```python
from build123d import *

# Parameters (mm, degrees)
SKETCH080_W         = 21.5
SKETCH080_H         = 41.5
PAD036_DEPTH        = 7
SKETCH081_W         = 17.5
SKETCH081_H         = 37.5
POCKET027_DEPTH     = 5
SKETCH077_W         = 13.5
SKETCH077_H         = 33.5
POCKET028_DEPTH     = 2.001
SKETCH078_W         = 13.5
SKETCH078_H         = 4
POCKET026_DEPTH     = 7.001
REVOLUTION010_ANGLE = -180
REVOLUTION011_ANGLE = -180


with BuildPart() as part:
    # Sketch080 → Pad036 (new body)
    with BuildSketch(Plane.XY):
        with Locations((10.75, 20.75)):
            Rectangle(SKETCH080_W, SKETCH080_H)
    extrude(amount=PAD036_DEPTH)

    # Sketch081 (on Face6 of Pad036) → Pocket027 (cut)
    with BuildSketch(Plane.XY.offset(7)):
        with Locations((10.75, 20.75)):
            Rectangle(SKETCH081_W, SKETCH081_H)
    extrude(amount=-POCKET027_DEPTH, mode=Mode.SUBTRACT)

    # Sketch077 (on Face11 of Pocket027) → Pocket028 (cut, through all)
    with BuildSketch(Plane.XY.offset(2)):
        with Locations((10.75, 20.75)):
            Rectangle(SKETCH077_W, SKETCH077_H)
    extrude(amount=-POCKET028_DEPTH, mode=Mode.SUBTRACT)

    # Sketch078 (on Face5 of Pocket028) → Pocket026 (cut, through all)
    with BuildSketch(Plane.XY.offset(7)):
        with Locations((10.75, 2)):
            Rectangle(SKETCH078_W, SKETCH078_H)
    extrude(amount=-POCKET026_DEPTH, mode=Mode.SUBTRACT)

    # Sketch082 (on Face18 of Pocket026) → Revolution010 (revolve)
    with BuildSketch(Plane.YZ.offset(2)):
        with BuildLine():
            ThreePointArc((7, 6), (6, 7), (5, 6))
            Line((5, 6), (7, 6))
        make_face()
        with BuildLine():
            ThreePointArc((36.5, 6), (35.5, 7), (34.5, 6))
            Line((34.5, 6), (36.5, 6))
        make_face()
    revolve(axis=Axis((2, 34.5, 6), (0, -1, 0)), revolution_arc=REVOLUTION010_ANGLE)

    # Sketch083 (on Face17 of Revolution010) → Revolution011 (revolve)
    with BuildSketch(Plane(origin=(19.5, 0, 0), x_dir=(0, -1, 0), z_dir=(-1, 0, 0))):
        with BuildLine():
            ThreePointArc((-34.5, 6), (-35.5, 7), (-36.5, 6))
            Line((-36.5, 6), (-34.5, 6))
        make_face()
        with BuildLine():
            ThreePointArc((-5, 6), (-6, 7), (-7, 6))
            Line((-7, 6), (-5, 6))
        make_face()
    revolve(axis=Axis((19.5, 7, 6), (0, 1, 0)), revolution_arc=REVOLUTION011_ANGLE)


solid = part.part
```
Here's how the part is built. I have some questions about the finished solid (model axes, mm). A direction names the side the tool comes from. Round coordinates to 2 decimals unless told otherwise and drop trailing zeros. Write each loop counter-clockwise with the first axis right and the second up, starting at its lowest first coordinate (ties: lowest second). Pieces come first, ordered by that corner, then holes. Notation, with made-up numbers: M -35,32 L -30,32 A28 cw -30,53 Z; hole C 80.25,78.25 d5. An arc over 180 degrees is marked long. Answer as CSV lines item,"result". Start each with the question number.
1. On a 3-axis mill with a long thin cutter (end or side, diameter ignored), from which of +Z, -Z, +X, -X, +Y, -Y can I reach the whole of each face in a straight line? I mean faces 4 (the flat face through (11, 37.5, 1)), 5 (the flat face through (3, 2, 5)), 6 (the flat face through (0, 20, 3)). Say none if no direction works.
2. Suppose I cut it at D-D on z = 4.5. Write out the boundary of the cut face in (x, y), then the cut area to 3 significant figures.
3. Suppose I cut it at B-B on z = 1.5. Write out the boundary of the cut face in (x, y).
4. Suppose I cut it at C-C on x = 16.5. Write out the boundary of the cut face in (y, z), then the cut area to 3 significant figures.
5. Suppose I cut it at A-A on y = 32. Write out the boundary of the cut face in (x, z), then the cut area to 3 significant figures.
6. I'm going to push flat-ended pins straight in: pin 1 Ø1 at (x, y) = (18.5, 12) entering from +Z; pin 2 Ø1 at (x, z) = (8.5, 1.5) entering from -Y; pin 3 Ø1.5 at (x, z) = (10.5, 4) entering from -Y. Where does each tip first touch, or does it pass through?
7. I need wall thicknesses on probe 1 along X at (y, z) = (10.5, 5.25); probe 2 along X at (y, z) = (32, 0.5); probe 3 along Y at (x, z) = (19, 6.5). Which ranges of each line are inside material? Lowest first, please.
8. Thinking about a two-plate mould opening in Y: for faces 1 (the flat face through (2, 0, 3)), 2 (the flat face through (19.5, 20, 5)), 3 (the flat face through (17.5, 14, 1)), which applies, released by +Y, released by -Y, zero draft, split by the parting line, or undercut?
Check result:
1,face 4,"+Z, -Z, -Y"
1,face 5,"+Z"
1,face 6,"+Z, -Z, -X, +Y, -Y"
2,outline,"M 0,0 L 4,0 L 4,2 L 2,2 L 2,39.5 L 19.5,39.5 L 19.5,2 L 17.5,2 L 17.5,0 L 21.5,0 L 21.5,41.5 L 0,41.5 Z"
2,area,"209 mm2"
3,outline,"M 0,0 L 4,0 L 4,37.5 L 17.5,37.5 L 17.5,0 L 21.5,0 L 21.5,41.5 L 0,41.5 Z"
4,outline,"M 37.5,0 L 41.5,0 L 41.5,7 L 39.5,7 L 39.5,2 L 37.5,2 Z"
4,area,"18.0 mm2"
5,outline,"M 0,0 L 4,0 L 4,2 L 2,2 L 2,7 L 0,7 Z; M 17.5,0 L 21.5,0 L 21.5,7 L 19.5,7 L 19.5,2 L 17.5,2 Z"
5,area,"36.0 mm2"
6,pin 1,"stops at z = 2"
6,pin 2,"stops at y = 37.5"
6,pin 3,"stops at y = 39.5"
7,probe 1,"x = 0 to 2, 19.5 to 21.5"
7,probe 2,"x = 0 to 4, 17.5 to 21.5"
7,probe 3,"y = 0 to 2, 5.29 to 6.71, 34.79 to 36.21, 39.5 to 41.5"
8,face 1,"released by -Y"
8,face 2,"undercut"
8,face 3,"zero draft"
